Part print with two shaded views. Sizes in mm from the minimum x, y, z corner. Give positions to 0.01 mm unless a question says otherwise; leave off trailing zeros. Write each loop counter-clockwise with the first axis right and the second up, starting at its lowest first coordinate (ties: lowest second). Pieces come first, ordered by that corner, then holes. Notation, with made-up numbers: (38.5, 21) - (86.5, 21) arc R19 cw to (86.5, 25) - close; hole circle Ø10 at (79, -40). An arc over 180 degrees is marked (long way). One line per item, written item: value. Start each with the question number.
(1) Drop flat-ended pins along their axis: P1, Ø12, axis at y = 105, z = 100.5, coming from the +X side; P2, Ø4, axis at y = 79, z = 117, coming from the -X side; P3, Ø5, axis at x = 215, z = 129.5, coming from the +Y side. Give the stop position or say it passes through.
(2) Cut at D-D, the plane y = 411.5. List the corners of the cut face in (x, z), and give its area (3 significant figures).
(3) Probe L1, parallel to Y at x = 150, z = 115; L2, parallel to Z at x = 16.5, y = 209; L3, parallel to Z at x = 131, y = 409. List the from-to ranges inside material, lowest first.
(4) Cut at B-B, the plane x = 150. List the corners of the cut face in (y, z), and give its area (3 significant figures).
(5) Mould opens along Z. For the marked faces 1, 2 and 3 say: pulls with the +Z half, pulls with the -Z half, needs draft (parallel to the pull), parting line crosses it, or undercut.
(6) Cut at C-C, the plane z = 126.5. List the corners of the cut face in (x, y).
(7) Cut at A-A, the plane y = 150. List the corners of the cut face in (x, z), and give its area (3 significant figures).
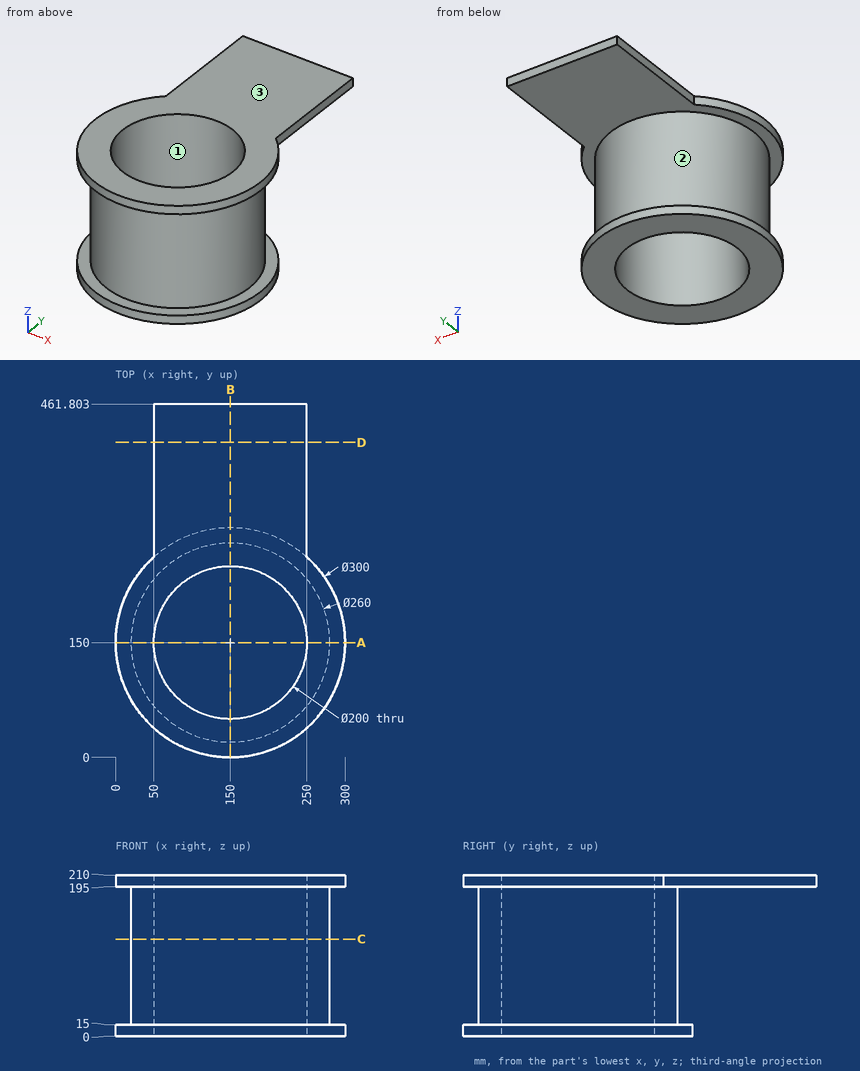
Answers follow:
1. P1: stops at x = 274.01
1. P2: stops at x = 39.82
1. P3: stops at y = 263.99
2. outline: (50, 195) - (250, 195) - (250, 210) - (50, 210) - close
2. area: 3,000 mm²
3. L1: y = 20 to 50, 250 to 280
3. L2: z = 0 to 15, 195 to 210
3. L3: z = 195 to 210
4. outline: (0, 0) - (50, 0) - (50, 210) - (0, 210) - (0, 195) - (20, 195) - (20, 15) - (0, 15) - close; (250, 0) - (300, 0) - (300, 15) - (280, 15) - (280, 195) - (461.8, 195) - (461.8, 210) - (250, 210) - close
4. area: 16,200 mm²
5. face 1: needs draft
5. face 2: undercut
5. face 3: pulls with the +Z half
6. outline: circle Ø260 at (150, 150); hole circle Ø200 at (150, 150)
7. outline: (0, 0) - (50, 0) - (50, 210) - (0, 210) - (0, 195) - (20, 195) - (20, 15) - (0, 15) - close; (250, 0) - (300, 0) - (300, 15) - (280, 15) - (280, 195) - (300, 195) - (300, 210) - (250, 210) - close
7. area: 13,800 mm²
